Source: CAD feature listing. Evaluate the final solid. Frame: model axes, mm. A direction names the side the tool comes from. Coordinates: 2 decimals unless noted, no trailing zeros. Order: outer loops, then holes, each group sorted by start corner. A loop starts at its lowest first (then second) coordinate and runs counter-clockwise, first axis right, second up. Notation, with made-up numbers: (-26, -3) -> (27, -3) arc R19 cw to (27, 6) -> close; hole circle Ø5 at (-12.75, -29.75). An arc over 180 degrees is marked (long way). Write item = value, one per line. Start each with the question number.
Item 1: Mould query, pull axis X, two halves, no side actions, for faces 1 (the flat face through (-124.1, -32, -27)), 2 (the flat face through (-122.1, -32, -30.9)), 3 (the flat face through (-114.4, -35.6, -26.1)), 4 (the flat face through (-126, -39, -1.5)). Classes: released by +X, released by -X, zero draft, split by the parting line, or undercut.
Item 2: Section query B-B (y = -40.75). Output: boundary loops of the cut face in (x, z), then the cut area to 3 significant figures.
Item 3: Contact query for flat-ended pins moving along their axis: pin 1 (2.5 mm diameter, centred on y = -32.5, z = -31.5, fed in from +X); pin 2 (8.5 mm diameter, centred on y = -34.5, z = -28, fed in from -X); pin 3 (2 mm diameter, centred on x = -123, z = -33, fed in from -Y). Output: stop coordinate, or through.
Item 4: Section query C-C (x = -127.5). Output: boundary loops of the cut face in (y, z).
Item 5: Section query A-A (z = -33). Output: boundary loops of the cut face in (x, y), then the cut area to 3 significant figures.
Item 6: Set-up query: faces 5 (the flat face through (-122, -27.9, -26)), 6 (the flat face through (-123, -32, -29.4)), 7 (the flat face through (-121.6, -27, -26)). Return all of +Z, -Z, +X, -X, +Y, -Y with unobstructed straight access to the full face (end or side cutting, diameter ignored); none if empty.
Item 7: Section query D-D (z = -23). Output: boundary loops of the cut face in (x, y), then the cut area to 3 significant figures.
Item 8: Ray query, line 1 along Z through (x, y) = (-127.25, -32.25); line 2 along X through (y, z) = (-28, -18.5); line 3 along Y through (x, z) = (-118.75, -43.5). Return the intervals inside material, ascending. Write a range as [from, to].
```python
from build123d import *

# Parameters (mm, degrees)
BOSS_EXTRUDE1_DEPTH = 52.5
BOSS_EXTRUDE2_DEPTH = 1.5
CUT_EXTRUDE1_REACH  = 73.793
SKETCH5_W           = 2
SKETCH5_H           = 4
BOSS_EXTRUDE3_DEPTH = 1
FILLET1_R           = 5
BOSS_EXTRUDE4_DEPTH = 1
CHAMFER3_SIZE       = 0.5
CHAMFER4_SIZE       = 1
FILLET3_R           = 0.5
FILLET4_R           = 0.5


with BuildPart() as part:
    # Sketch1 → Boss-Extrude1 (new body)
    with BuildSketch(Plane.XY):
        Polygon((-121.6, -26.1), (-124.1, -26.1), (-124.1, -37.6), (-112.6, -37.6), (-112.6, -35.1), (-114.4, -35.1), (-114.4, -36.1), (-122.6, -36.1), (-122.6, -27.9), (-121.6, -27.9), align=None)
    extrude(amount=-BOSS_EXTRUDE1_DEPTH)

    # Sketch2 → Boss-Extrude2 (add)
    with BuildSketch(Plane.XY):
        Polygon((-124.1, -26.1), (-134.1, -26.1), (-134.1, -47.6), (-112.6, -47.6), (-112.6, -37.6), (-124.1, -37.6), align=None)
    extrude(amount=-BOSS_EXTRUDE2_DEPTH)

    # Sketch4 → Cut-Extrude1 (cut, up to next)
    with BuildSketch(Plane(origin=(-122.6, 0, 0), x_dir=(0, 0, -1), z_dir=(1, 0, 0)), mode=Mode.PRIVATE) as cut_extrude1_sk1:
        Polygon((36.4, -30), (36.4, -29), (28.4, -29), (28.4, -35), (36.4, -35), (36.4, -34), (29.4, -34), (29.4, -30), align=None)
    cut_extrude1_tool1 = extrude(cut_extrude1_sk1.sketch, amount=-CUT_EXTRUDE1_REACH, mode=Mode.PRIVATE) & part.part
    add(cut_extrude1_tool1.solids().sort_by_distance((-122.6, -29.5, -36.3))[0], mode=Mode.SUBTRACT)

    # Sketch5 → Boss-Extrude3 (add)
    with BuildSketch(Plane(origin=(-122.6, 0, 0), x_dir=(0, 0, -1), z_dir=(1, 0, 0))):
        with Locations((30.4, -32)):
            Rectangle(SKETCH5_W, SKETCH5_H)
    extrude(amount=BOSS_EXTRUDE3_DEPTH)

    # Fillet1
    fillet1_edges = [part.edges().sort_by_distance(p)[0] for p in [
        (-112.6, -47.6, -0.75),
        (-134.1, -47.6, -0.75),
        (-134.1, -26.1, -0.75),
    ]]
    fillet(fillet1_edges, radius=FILLET1_R)

    # Sketch6 → Boss-Extrude4 (add)
    with BuildSketch(Plane(origin=(0, 0, -52.5), x_dir=(-1, 0, 0), z_dir=(0, 0, -1))):
        Polygon((112.6, -35.1), (112.6, -37.6), (124.1, -37.6), (124.1, -26.1), (121.6, -26.1), align=None)
    extrude(amount=BOSS_EXTRUDE4_DEPTH)

    # Chamfer3
    chamfer3_edges = [part.edges().sort_by_distance(p)[0] for p in [
        (-118.5, -36.1, 0),
        (-114.4, -35.6, 0),
        (-117.1, -30.6, -53.5),
        (-113.5, -35.1, 0),
        (-112.6, -36.35, -53.5),
        (-118.35, -37.6, -53.5),
        (-124.1, -31.85, -53.5),
        (-122.85, -26.1, -53.5),
        (-125.35, -26.1, 0),
        (-121.6, -27, 0),
        (-134.1, -36.85, 0),
        (-123.35, -47.6, 0),
        (-112.6, -38.85, 0),
        (-114.064466094, -46.135533906, 0),
        (-132.635533906, -46.135533906, 0),
        (-132.635533906, -27.564466094, 0),
        (-122.1, -27.9, 0),
        (-122.6, -32, 0),
    ]]
    chamfer(chamfer3_edges, length=CHAMFER3_SIZE)

    # Chamfer4
    chamfer4_edges = [part.edges().sort_by_distance(p)[0] for p in [
        (-121.6, -32, -31.4),
        (-121.6, -32, -29.4),
    ]]
    chamfer(chamfer4_edges, length=CHAMFER4_SIZE - 0.0001)  # a hair under: the kernel refuses the full size

    # Fillet3
    fillet3_edges = [part.edges().sort_by_distance(p)[0] for p in [
        (-123.35, -29, -36.4),
        (-123.35, -30, -36.4),
        (-123.35, -34, -36.4),
        (-123.35, -35, -36.4),
    ]]
    fillet(fillet3_edges, radius=FILLET3_R - 0.0001)  # a hair under: the kernel refuses the full size

    # Fillet4
    fillet4_edges = [part.edges().sort_by_distance(p)[0] for p in [
        (-124.1, -26.1, -27.25),
        (-124.1, -37.6, -27.25),
        (-112.6, -37.6, -27.25),
    ]]
    fillet(fillet4_edges, radius=FILLET4_R)


solid = part.part
```
Computed:
q1.face_1 = released by -X
q1.face_2 = released by +X
q1.face_3 = undercut
q1.face_4 = zero draft
q2.outline = (-134.1, -1.5) -> (-112.6, -1.5) -> (-112.6, -0.5) -> (-113.1, 0) -> (-133.6, 0) -> (-134.1, -0.5) -> close
q2.area = 32.0 mm^2
q3.pin_1 = -121.6
q3.pin_2 = -124.1
q3.pin_3 = -37.6
q4.outline = (-47.6, -1.5) -> (-26.1, -1.5) -> (-26.1, -0.5) -> (-26.6, 0) -> (-47.1, 0) -> (-47.6, -0.5) -> close
q5.outline = (-124.1, -37.1) arc R0.5 ccw to (-123.6, -37.6) -> (-113.1, -37.6) arc R0.5 ccw to (-112.6, -37.1) -> (-112.6, -35.1) -> (-114.4, -35.1) -> (-114.4, -36.1) -> (-122.6, -36.1) -> (-122.6, -35) -> (-124.1, -35) -> close; (-124.1, -34) -> (-122.6, -34) -> (-122.6, -30) -> (-124.1, -30) -> close; (-124.1, -29) -> (-122.6, -29) -> (-122.6, -27.9) -> (-121.6, -27.9) -> (-121.6, -26.1) -> (-123.6, -26.1) arc R0.5 ccw to (-124.1, -26.6) -> close
q5.area = 32.7 mm^2
q6.face_5 = +Z, +X
q6.face_6 = +X, -X
q6.face_7 = +Z, +X, +Y
q7.outline = (-124.1, -37.1) arc R0.5 ccw to (-123.6, -37.6) -> (-113.1, -37.6) arc R0.5 ccw to (-112.6, -37.1) -> (-112.6, -35.1) -> (-114.4, -35.1) -> (-114.4, -36.1) -> (-122.6, -36.1) -> (-122.6, -27.9) -> (-121.6, -27.9) -> (-121.6, -26.1) -> (-123.6, -26.1) arc R0.5 ccw to (-124.1, -26.6) -> close
q7.area = 35.7 mm^2
q8.line_1 = [-1.5, 0]
q8.line_2 = [-124.1, -122.6]
q8.line_3 = [-37.6, -36.1]
